Autodesk Inventor part; units mm, degrees
ref_plane "YZ Plane" through (0, 0, 0) normal (1, 0, 0) x (0, 1, 0)
ref_plane "XZ Plane" through (0, 0, 0) normal (0, 1, 0) x (-1, 0, 0)
ref_plane "XY Plane" through (0, 0, 0) normal (0, 0, 1) x (1, 0, 0)
sketch "Sketch1" plane through (0, 0, 0) normal (0, 0, 1) x (1, 0, 0)
  circle A0 centre (0, 0) radius 9
  circle A1 centre (0, 5) radius 1.5
  line L0 (1.4145, 2.45) -> (2.829, 0)
  line L1 (2.829, 0) -> (1.4145, -2.45)
  line L2 (1.4145, -2.45) -> (-1.4145, -2.45)
  line L3 (-1.4145, -2.45) -> (-2.829, 0)
  line L4 (-2.829, 0) -> (-1.4145, 2.45)
  line L5 (-1.4145, 2.45) -> (1.4145, 2.45)
  dimension "d0" = 18
  dimension "d1" = 4.9
  dimension "d2" = 5
  dimension "d3" = 3
extrude "Extrusion1" add sketch "Sketch1" against normal blind 3
properties part number "OutputDisk2"
Model file for the job. Use its own axes, mm. A direction names the side the tool comes from. Give positions to 0.01 mm unless a question says otherwise; leave off trailing zeros. Loops run counter-clockwise (first coordinate to the right, second up) from the corner with the lowest first, then second, coordinate; pieces in that order, holes last. Notation, with made-up numbers: (6.5, 71) -> (54.5, 71) arc R26 ccw to (54.5, 110) -> close; hole circle Ø10 at (0, 66). An arc over 180 degrees is marked (long way). Use a Markdown table: item, result. Add a question column.
(1) Slice it at A-A on z = -1.25. List the corners of the cut face in (x, y), and give its area (3 significant figures).
(2) Slice it at C-C on y = 5. List the corners of the cut face in (x, z), and give its area (3 significant figures).
(3) Mould opens along X. For faces 3 (the flat face through (-2.112, -1.242, -1.479)), 4 (the cylindrical face through (-1.172, 8.923, -1.479)), 5 (the flat face through (2, -2, 0)) say: +X half, -X half, draft (parallel to the pull), parting line (faces both ways), or undercut.
(4) Slice it at D-D on x = -3.5. List the corners of the cut face in (y, z).
(5) Tool access for faces 1 (the flat face through (2, -2, -3)), 2 (the flat face through (0, -2.45, -1)): list every direction of +Z, -Z, +X, -X, +Y, -Y with a clear straight run to the whole face (end or side of a thin tool).
(6) Wall check: line 1 along Y through (x, z) = (0, -1.7); line 2 along Y through (x, z) = (-0.75, -1.5); line 3 along X through (y, z) = (4.5, -2.05). Give the ranges that are in metal, low to high.
(7) Slice it at B-B on x = 0. List the corners of the cut face in (y, z).
Filled sheet:
| question | item | result |
|---|---|---|
| 1 | outline | circle Ø18 at (0, 0); hole (-2.83, 0) -> (-1.41, -2.45) -> (1.41, -2.45) -> (2.83, 0) -> (1.41, 2.45) -> (-1.41, 2.45) -> close; hole circle Ø3 at (0, 5) |
| 1 | area | 227 mm2 |
| 2 | outline | (-7.48, -3) -> (-1.5, -3) -> (-1.5, 0) -> (-7.48, 0) -> close; (1.5, -3) -> (7.48, -3) -> (7.48, 0) -> (1.5, 0) -> close |
| 2 | area | 35.9 mm2 |
| 3 | face 3 | undercut |
| 3 | face 4 | parting line |
| 3 | face 5 | draft |
| 4 | outline | (-8.29, -3) -> (8.29, -3) -> (8.29, 0) -> (-8.29, 0) -> close |
| 5 | face 1 | -Z, +X, -X, +Y, -Y |
| 5 | face 2 | +Z, -Z |
| 6 | line 1 | -9 to -2.45, 2.45 to 3.5, 6.5 to 9 |
| 6 | line 2 | -8.97 to -2.45, 2.45 to 3.7, 6.3 to 8.97 |
| 6 | line 3 | -7.79 to -1.41, 1.41 to 7.79 |
| 7 | outline | (-9, -3) -> (-2.45, -3) -> (-2.45, 0) -> (-9, 0) -> close; (2.45, -3) -> (3.5, -3) -> (3.5, 0) -> (2.45, 0) -> close; (6.5, -3) -> (9, -3) -> (9, 0) -> (6.5, 0) -> close |
